Verification items for the finished model (mm, model axes). A direction names the side the tool comes from. Give positions to 0.01 mm unless a question says otherwise; leave off trailing zeros. Loops run counter-clockwise (first coordinate to the right, second up) from the corner with the lowest first, then second, coordinate; pieces in that order, holes last. Notation, with made-up numbers: M 21,-18 L 75,-18 A13 ccw 75,-13 Z; hole C 70,43 d1. An arc over 180 degrees is marked long. Use a Markdown table: item, result.
from build123d import *

# Parameters (mm, degrees)
SKETCH1_R           = 13.5
BOSS_EXTRUDE1_DEPTH = 35
SKETCH2_R           = 12.5
BOSS_EXTRUDE2_DEPTH = 300
SHELL1_START        = -35
SHELL1_OUTLINE_R    = 12.5
SHELL1_DEPTH        = 70
SHELL1_2_OUTLINE_W  = 11.5
SHELL1_2_OUTLINE_H  = 295.102396758


with BuildPart() as part:
    # Sketch1 → Boss-Extrude1 (new, symmetric)
    with BuildSketch(Plane(origin=(0, 0, 0), x_dir=(1, 0, 0), z_dir=(0, 1, 0))):
        with Locations(Location((0, 0, 0), (0, 0, 270))):
            Circle(SKETCH1_R)
    extrude(amount=BOSS_EXTRUDE1_DEPTH, both=True)

    # Sketch2 → Boss-Extrude2 (add)
    with BuildSketch(Plane.XY):
        with Locations(Location((0, 0, 0), (0, 0, 180))):
            Circle(SKETCH2_R)
    extrude(amount=BOSS_EXTRUDE2_DEPTH)

    # Shell1: read off the stored shape, not the designer's step
    # Shell1 outline → Shell1 (cut)
    with BuildSketch(Plane(origin=(0, 0, 0), x_dir=(1, 0, 0), z_dir=(0, 1, 0)).offset(SHELL1_START)):
        Circle(SHELL1_OUTLINE_R)
    extrude(amount=SHELL1_DEPTH, mode=Mode.SUBTRACT)

    # Shell1 2 outline → Shell1 2 (revolve, cut)
    with BuildSketch(Plane.XZ):
        with Locations((5.75, 152.448801621)):
            Rectangle(SHELL1_2_OUTLINE_W, SHELL1_2_OUTLINE_H)
    revolve(axis=Axis((0, 0, 0), (0, 0, 1)), mode=Mode.SUBTRACT)


solid = part.part
(1) Cross-section at C-C on y = 0. Record the cut outline in (x, z), then the cut area to 3 significant figures.
Results below:
| item | result |
|---|---|
| outline | M -12.5,5.1 A13.5 ccw long 12.5,5.1 L 12.5,300 L 11.5,300 L 11.5,4.9 A12.5 cw long -11.5,4.9 L -11.5,300 L -12.5,300 Z |
| area | 641 mm^2 |
(2) Draft check along Y on faces 3 (the cylindrical face through (-1.5, 11.4, 154.5)), 4 (the flat face through (-9, 35, 9)), 5 (the cylindrical face through (-11.923, -3.755, 150.485)). Enter one of: +Y half, -Y half, draft (parallel to the pull), parting line (faces both ways), or undercut.
Results below:
| item | result |
|---|---|
| face 3 | undercut |
| face 4 | +Y half |
| face 5 | parting line |
(3) Cross-section at D-D on z = 272.5. Record the cut outline in (x, y), then the cut area to 3 significant figures.
Results below:
| item | result |
|---|---|
| outline | C 0,0 d25; hole C 0,0 d23 |
| area | 75.4 mm^2 |
(4) Cross-section at A-A on x = 0. Record the cut outline in (y, z), then the cut area to 3 significant figures.
Results below:
| item | result |
|---|---|
| outline | M -35,-13.5 L 35,-13.5 L 35,-12.5 L -35,-12.5 Z; M -35,12.5 L -11.5,12.5 L -11.5,300 L -12.5,300 L -12.5,13.5 L -35,13.5 Z; M 11.5,12.5 L 35,12.5 L 35,13.5 L 12.5,13.5 L 12.5,300 L 11.5,300 Z |
| area | 690 mm^2 |
(5) Gauge pin test, flat ends, axial feed: P1, Ø4, axis at x = -4, z = 206.5, coming from the +Y side; P2, Ø12, axis at x = -6.5, y = -3, coming from the -Z side; P3, Ø12, axis at x = -5, z = 147, coming from the +Y side. Record the tip position at first contact, or that the pin passes through.
Results below:
| item | result |
|---|---|
| P1 | y = 12.34 |
| P2 | z = -13.49 |
| P3 | y = 12.5 |
(6) Material ranges on line 1 (Y direction, x = -0.75, z = 202.5); line 2 (Z direction, x = -1, y = 32); line 3 (X direction, y = -5, z = 0), recorded low to high.
Results below:
| item | result |
|---|---|
| line 1 | -12.48 to -11.48, 11.48 to 12.48 |
| line 2 | -13.46 to -12.46, 12.46 to 13.46 |
| line 3 | -13.5 to -12.5, 12.5 to 13.5 |
(7) Cross-section at B-B on z = 0. Record the cut outline in (x, y).
Results below:
| item | result |
|---|---|
| outline | M -13.5,-35 L -12.5,-35 L -12.5,35 L -13.5,35 Z; M 12.5,-35 L 13.5,-35 L 13.5,35 L 12.5,35 Z |
(8) Set-up check for faces 1 (the cylindrical face through (0.594, 0.49, -13.487)), 2 (the flat face through (-9, -35, 9)): record each of +Z, -Z, +X, -X, +Y, -Y from which the full face is reachable in a straight line by a thin tool's end or side.
Results below:
| item | result |
|---|---|
| face 1 | none |
| face 2 | +Z, -Z, +X, -X, -Y |
